Work out the finished part from the listing and answer in its coordinate system (mm). Give positions to 0.01 mm unless a question says otherwise; leave off trailing zeros. Order: outer loops, then holes, each group sorted by start corner. A loop starts at its lowest first (then second) coordinate and runs counter-clockwise, first axis right, second up. Notation, with made-up numbers: (65.5, -20.75) -> (120.5, -20.75) arc R24 cw to (120.5, -7.75) -> close; hole circle Ø5 at (-13, 23). An arc over 180 degrees is marked (long way). Answer as CSV lines item,"result". Start each with the question number.
1. A cutting plane is placed at C-C (z = -10.5). Give the vertices of the cut face in (x, y), then the cut area to 3 significant figures.
2. A cutting plane is placed at D-D (y = 21.35). State how many separate pieces and enclosed holes the cut face has, then the cut area to 3 significant figures.
3. Find the intervals of material crossed by L1, parallel to X at y = 20.9, z = -11.25; L2, parallel to Z at x = 11.25, y = 20.7; L3, parallel to Z at x = 6, y = 21.5, in increasing order.
4. Flat-ended cylindrical pins translate along their axes: pin 1 (2.5 mm diameter, centred on x = 6, z = 6, fed in from +Y); pin 2 (4 mm diameter, centred on x = -6, z = 6, fed in from -Y); pin 3 (1 mm diameter, centred on x = -9, y = 21, fed in from +Z). Find the tip coordinate at first contact, or state that the pin passes through.
5. A cutting plane is placed at A-A (z = 0). Give the vertices of the cut face in (x, y), then the cut area to 3 significant figures.
6. A cutting plane is placed at B-B (x = -1.5). Give the vertices of the cut face in (y, z), then the cut area to 3 significant figures.
from build123d import *

# Parameters (mm, degrees)
CYLINDER006_R              = 1.45
CYLINDER006_DEPTH          = 10
CYLINDER007_R              = 1.45
CYLINDER007_DEPTH          = 10
CYLINDER008_R              = 1.45
CYLINDER008_DEPTH          = 10
CYLINDER009_R              = 1.45
CYLINDER009_DEPTH          = 10
CYLINDER005_R              = 1.45
CYLINDER005_DEPTH          = 10
CYLINDER002_R              = 1.45
CYLINDER002_DEPTH          = 10
CYLINDER003_R              = 1.45
CYLINDER003_DEPTH          = 10
CYLINDER004_R              = 1.45
CYLINDER004_DEPTH          = 10
CYLINDER001_R              = 4.5
CYLINDER001_DEPTH          = 10
CYLINDER_R                 = 7.5
CYLINDER_DEPTH             = 15
BOX001_W                   = 20
BOX001_H                   = 20
BOX001_DEPTH               = 10
BOX001_PLACEMENT_ANGLE     = 45
BOX002_W                   = 20
BOX002_H                   = 20
BOX002_DEPTH               = 10
BOX002_PLACEMENT_ANGLE     = 45
CLONE_PLACEMENT_ANGLE      = 90
BOX_W                      = 30
BOX_H                      = 30
BOX_DEPTH                  = 2
FILLET_R                   = 3.75
FILLET001_R                = 3.5
CUT010_PLACEMENT_ANGLE     = 90
CHAMFER004_SIZE            = 1
CHAMFER004_PLACEMENT_ANGLE = 180


with BuildPart() as cylinder006:
    # Cylinder006 → Cylinder006 (new body)
    with BuildSketch(Plane(origin=(11.25, -11.25, 0), x_dir=(1, 0, 0), z_dir=(0, 0, 1))):
        Circle(CYLINDER006_R)
    extrude(amount=CYLINDER006_DEPTH)


with BuildPart() as cylinder007:
    # Cylinder007 → Cylinder007 (new body)
    with BuildSketch(Plane(origin=(11.25, 11.25, 0), x_dir=(1, 0, 0), z_dir=(0, 0, 1))):
        Circle(CYLINDER007_R)
    extrude(amount=CYLINDER007_DEPTH)


with BuildPart() as cylinder008:
    # Cylinder008 → Cylinder008 (new body)
    with BuildSketch(Plane(origin=(-11.25, -11.25, 0), x_dir=(1, 0, 0), z_dir=(0, 0, 1))):
        Circle(CYLINDER008_R)
    extrude(amount=CYLINDER008_DEPTH)


with BuildPart() as cylinder009:
    # Cylinder009 → Cylinder009 (new body)
    with BuildSketch(Plane(origin=(-11.25, 11.25, 0), x_dir=(1, 0, 0), z_dir=(0, 0, 1))):
        Circle(CYLINDER009_R)
    extrude(amount=CYLINDER009_DEPTH)


with BuildPart() as cylinder005:
    # Cylinder005 → Cylinder005 (new body)
    with BuildSketch(Plane(origin=(6, -6, 0), x_dir=(1, 0, 0), z_dir=(0, 0, 1))):
        Circle(CYLINDER005_R)
    extrude(amount=CYLINDER005_DEPTH)


with BuildPart() as cylinder002:
    # Cylinder002 → Cylinder002 (new body)
    with BuildSketch(Plane(origin=(6, 6, 0), x_dir=(1, 0, 0), z_dir=(0, 0, 1))):
        Circle(CYLINDER002_R)
    extrude(amount=CYLINDER002_DEPTH)


with BuildPart() as cylinder003:
    # Cylinder003 → Cylinder003 (new body)
    with BuildSketch(Plane(origin=(-6, 6, 0), x_dir=(1, 0, 0), z_dir=(0, 0, 1))):
        Circle(CYLINDER003_R)
    extrude(amount=CYLINDER003_DEPTH)


with BuildPart() as cylinder004:
    # Cylinder004 → Cylinder004 (new body)
    with BuildSketch(Plane(origin=(-6, -6, 0), x_dir=(1, 0, 0), z_dir=(0, 0, 1))):
        Circle(CYLINDER004_R)
    extrude(amount=CYLINDER004_DEPTH)


with BuildPart() as cylinder001:
    # Cylinder001 → Cylinder001 (new body)
    with BuildSketch(Plane.XY):
        Circle(CYLINDER001_R)
    extrude(amount=CYLINDER001_DEPTH)


with BuildPart() as cylinder:
    # Cylinder → Cylinder (new body)
    with BuildSketch(Plane.XY):
        Circle(CYLINDER_R)
    extrude(amount=CYLINDER_DEPTH)


with BuildPart() as cube001:
    # Box001 → Box001 (new body)
    with BuildSketch(Plane.XY):
        with Locations((10, 10)):
            Rectangle(BOX001_W, BOX001_H)
    extrude(amount=BOX001_DEPTH)


with BuildPart() as cube001_1:
    # Box001 placement: moved
    add(cube001.part.moved(Location((0, -33.53, 0))).rotate(Axis((0, -33.53, 0), (0, 0, 1)), BOX001_PLACEMENT_ANGLE))


with BuildPart() as cut:
    # Box002 → Box002 (new body)
    with BuildSketch(Plane.XY):
        with Locations((10, 10)):
            Rectangle(BOX002_W, BOX002_H)
    extrude(amount=BOX002_DEPTH)


with BuildPart() as cut_1:
    # Box002 placement: moved
    add(cut.part.moved(Location((0, 5.35, 0))).rotate(Axis((0, 5.35, 0), (0, 0, 1)), BOX002_PLACEMENT_ANGLE))

    # Fusion: union Cube001
    add(cube001_1.part)

    # Cut: cut Cylinder
    add(cylinder.part, mode=Mode.SUBTRACT)


with BuildPart() as cut001:
    # Clone base: copy of Cut
    add(cut_1.part)


with BuildPart() as cut001_1:
    # Clone placement: moved
    add(cut001.part.rotate(Axis((0, 0, 0), (0, 0, 1)), CLONE_PLACEMENT_ANGLE))


with BuildPart() as fusion001:
    # Fusion001 base: copy of Cut
    add(cut_1.part)

    # Fusion001: union Cut001
    add(cut001_1.part)


with BuildPart() as obj1:
    # Box → Box (new body)
    with BuildSketch(Plane(origin=(-15, -15, 0), x_dir=(1, 0, 0), z_dir=(0, 0, 1))):
        with Locations((15, 15)):
            Rectangle(BOX_W, BOX_H)
    extrude(amount=BOX_DEPTH)

    # Fillet
    fillet_edges = [obj1.edges().sort_by_distance(p)[0] for p in [
        (-15, -15, 1),
        (-15, 15, 1),
        (15, -15, 1),
        (15, 15, 1),
    ]]
    fillet(fillet_edges, radius=FILLET_R)

    # Cut001: cut Fusion001
    add(fusion001.part, mode=Mode.SUBTRACT)

    # Fillet001
    fillet001_edges = [obj1.edges().sort_by_distance(p)[0] for p in [
        (-15, -9.65, 1),
        (-15, 9.65, 1),
        (-9.65, 15, 1),
        (9.65, 15, 1),
        (15, 9.754271, 1),
        (15, -9.754271, 1),
        (9.754271, -15, 1),
        (-9.754271, -15, 1),
    ]]
    fillet(fillet001_edges, radius=FILLET001_R)

    # Cut002: cut Cylinder001
    add(cylinder001.part, mode=Mode.SUBTRACT)

    # Cut003: cut Cylinder004
    add(cylinder004.part, mode=Mode.SUBTRACT)

    # Cut004: cut Cylinder003
    add(cylinder003.part, mode=Mode.SUBTRACT)

    # Cut005: cut Cylinder002
    add(cylinder002.part, mode=Mode.SUBTRACT)

    # Cut006: cut Cylinder005
    add(cylinder005.part, mode=Mode.SUBTRACT)

    # Cut007: cut Cylinder009
    add(cylinder009.part, mode=Mode.SUBTRACT)

    # Cut008: cut Cylinder008
    add(cylinder008.part, mode=Mode.SUBTRACT)

    # Cut009: cut Cylinder007
    add(cylinder007.part, mode=Mode.SUBTRACT)

    # Cut010: cut Cylinder006
    add(cylinder006.part, mode=Mode.SUBTRACT)


with BuildPart() as obj1_1:
    # Cut010 placement: moved
    add(obj1.part.rotate(Axis((0, 0, 0), (1, 0, 0)), CUT010_PLACEMENT_ANGLE))

    # Chamfer004
    chamfer004_edges = [obj1_1.edges().sort_by_distance(p)[0] for p in [
        (4.55, 0, 6),
        (-7.45, 0, 6),
        (4.55, 0, -6),
        (-7.45, 0, -6),
    ]]
    chamfer(chamfer004_edges, length=CHAMFER004_SIZE)


with BuildPart() as obj1_2:
    # Chamfer004 placement: moved
    add(obj1_1.part.moved(Location((0, 20, 0))).rotate(Axis((0, 20, 0), (1, 0, 0)), CHAMFER004_PLACEMENT_ANGLE))


solid = obj1_2.part
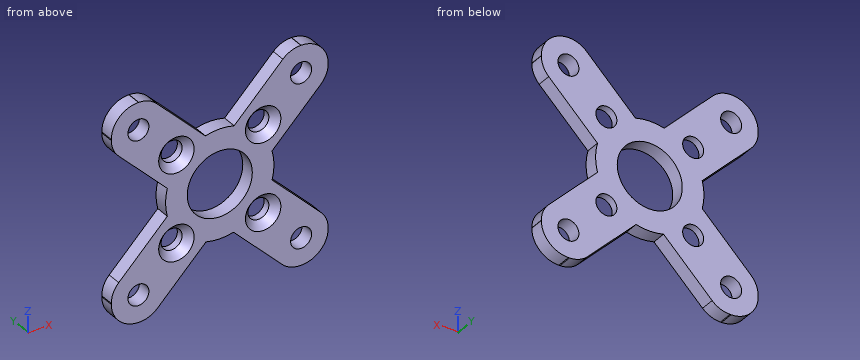
Answer sheet:
1,outline,"(-14.95, 20) -> (-12.49, 20) -> (-12.49, 22) -> (-14.95, 22) -> close; (-10.01, 20) -> (-5.15, 20) -> (-5.15, 22) -> (-10.01, 22) -> close; (5.15, 20) -> (10.01, 20) -> (10.01, 22) -> (5.15, 22) -> close; (12.49, 20) -> (14.93, 20) -> (14.93, 22) -> (12.49, 22) -> close"
1,area,"29.2 mm^2"
2,separate pieces,"1"
2,enclosed holes,"9"
2,area,"411 mm^2"
3,L1,"x = -15 to -12.7, -9.8 to -5.9, 5.9 to 9.8, 12.7 to 15"
3,L2,"z = -15 to -12.7, -9.8 to -6, 6 to 9.8, 12.7 to 15"
3,L3,"z = -11.35 to -7.45, -4.55 to 4.55, 7.45 to 11.25"
4,pin 1,"passes through"
4,pin 2,"stops at y = 20.45"
4,pin 3,"stops at z = 14.56"
5,outline,"(-7.5, 20) -> (-4.5, 20) -> (-4.5, 22) -> (-7.5, 22) -> close; (4.5, 20) -> (7.5, 20) -> (7.5, 22) -> (4.5, 22) -> close"
5,area,"12.0 mm^2"
6,outline,"(20, -7.35) -> (22, -7.35) -> (22, -4.24) -> (20, -4.24) -> close; (20, 4.24) -> (22, 4.24) -> (22, 7.35) -> (20, 7.35) -> close"
6,area,"12.4 mm^2"
